Source: CAD feature listing. Evaluate the final solid. Frame: model axes, mm. Face numbers are marked on the shaded views. A direction names the side the tool comes from. Round coordinates to 2 decimals unless told otherwise and drop trailing zeros. Order: outer loops, then holes, each group sorted by start corner. A loop starts at its lowest first (then second) coordinate and runs counter-clockwise, first axis right, second up. Notation, with made-up numbers: (-24.75, -18.5) -> (28.25, -18.5) arc R7 cw to (28.25, -7.5) -> close; hole circle Ø5 at (2, 11). An arc over 180 degrees is marked (long way). Write item = value, one per line. Start each with the question number.
(1) Ray query, line 1 (Y direction, x = 30, z = 14.5); line 2 (Y direction, x = 30, z = 6); line 3 (Y direction, x = 0.5, z = 3). Return the intervals inside material, ascending.
(2) Contact query for flat-ended pins moving along their axis: pin 1 Ø9.5 at (x, y) = (0.5, -1.5) entering from +Z; pin 2 Ø10.5 at (x, y) = (-30, -30) entering from +Z; pin 3 Ø4 at (x, z) = (29, 38.5) entering from -Y; pin 4 Ø9 at (x, y) = (30, -30) entering from -Z. Output: stop coordinate, or through.
(3) Cut plane C-C on x = 30. Return the cut outline in (y, z), then the cut area to 3 significant figures.
(4) Draft query along Y for the marked faces 1, 2, 3 and 4. Return one class per face: released by +Y, released by -Y, zero draft, split by the parting line, or undercut.
(5) Cut plane D-D on y = 11. Return the cut outline in (x, z).
(6) Reachability of the marked faces 5, 6 and 7 from +Z, -Z, +X, -X, +Y, -Y: full face, straight path, thin tool, end or side. Return the list, or none.
(7) Cut plane A-A on y = 30. Return the cut outline in (x, z).
(8) Cut plane B-B on z = 9.5. Give the number of separate pieces and of enclosed holes in the cut face, then the cut area to 3 significant figures.
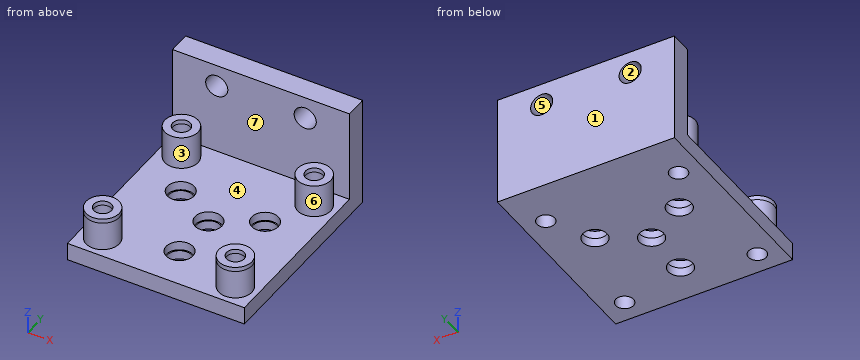
from build123d import *

# Parameters (mm, degrees)
F0_W      = 80
F0_H      = 80
F1_DEPTH  = 8
F2_R      = 6.05
F2_R_2    = 5.5
F3_DEPTH  = 4
F4_DEPTH  = 25
F5_DEPTH  = 25
F6_R      = 7.5
F6_R_2    = 4
F7_DEPTH  = 13
F8_DEPTH  = 25
F9_W      = 80
F9_H      = 10
F10_DEPTH = 50
F11_R     = 5
F12_DEPTH = 25
F13_DEPTH = 2


with BuildPart() as f1:
    # F0 (on Top) → F1 (new body)
    with BuildSketch(Plane.XY):
        Rectangle(F0_W, F0_H)
    extrude(amount=F1_DEPTH)

    # F2 (on face) → F3 (cut)
    with BuildSketch(Plane.XY.offset(8)):
        with Locations((-19.0525588833, 11)):
            Circle(F2_R)
        with Locations((-19.0525588833, 11)):
            Circle(F2_R_2, mode=Mode.SUBTRACT)
        with Locations((19.0525588833, 11)):
            Circle(F2_R)
        with Locations((19.0525588833, 11)):
            Circle(F2_R_2, mode=Mode.SUBTRACT)
        Circle(F2_R)
        Circle(F2_R_2, mode=Mode.SUBTRACT)
        with Locations((0, -22)):
            Circle(F2_R)
        with Locations((0, -22)):
            Circle(F2_R_2, mode=Mode.SUBTRACT)
    extrude(amount=-F3_DEPTH, mode=Mode.SUBTRACT)

    # F4 (cut): faces of the model
    f4_faces = [f1.faces().sort_by_distance(p)[0] for p in [
        (-19.0525588833, 11, 8),
        (19.0525588833, 11, 8),
        (0, -22, 8),
    ]]
    extrude(f4_faces, amount=-F4_DEPTH, mode=Mode.SUBTRACT)

    # F5 (cut): a face of the model
    f5_faces = [f1.faces().sort_by_distance(p)[0] for p in [
        (0, 0, 8),
    ]]
    extrude(f5_faces, amount=-F5_DEPTH, mode=Mode.SUBTRACT)

    # F6 (on face) → F7 (join)
    with BuildSketch(Plane.XY.offset(8)):
        with Locations((-30, 30)):
            Circle(F6_R)
        with Locations((-30, 30)):
            Circle(F6_R_2, mode=Mode.SUBTRACT)
        with Locations((30, 30)):
            Circle(F6_R)
        with Locations((30, 30)):
            Circle(F6_R_2, mode=Mode.SUBTRACT)
        with Locations((30, -30)):
            Circle(F6_R)
        with Locations((30, -30)):
            Circle(F6_R_2, mode=Mode.SUBTRACT)
        with Locations((-30, -30)):
            Circle(F6_R)
        with Locations((-30, -30)):
            Circle(F6_R_2, mode=Mode.SUBTRACT)
    extrude(amount=F7_DEPTH)

    # F8 (cut): faces of the model
    f8_faces = [f1.faces().sort_by_distance(p)[0] for p in [
        (-30, 30, 8),
        (30, 30, 8),
        (-30, -30, 8),
        (30, -30, 8),
    ]]
    extrude(f8_faces, amount=-F8_DEPTH, mode=Mode.SUBTRACT)

    # F9 (on face) → F10 (join)
    with BuildSketch(Plane(origin=(0, 0, 0), x_dir=(1, 0, 0), z_dir=(0, 0, -1))):
        with Locations((0, -45)):
            Rectangle(F9_W, F9_H)
    extrude(amount=-F10_DEPTH)

    # F11 (on face) → F12 (cut)
    with BuildSketch(Plane(origin=(0, 50, 0), x_dir=(-1, 0, 0), z_dir=(0, 1, 0))):
        with Locations((-20, 40)):
            Circle(F11_R)
        with Locations((20, 40)):
            Circle(F11_R)
    extrude(amount=-F12_DEPTH, mode=Mode.SUBTRACT)

    # F13 (add): faces of the model
    f13_faces = [f1.faces().sort_by_distance(p)[0] for p in [
        (-37.2878679656, 30, 21),
        (-37.2878679656, -30, 21),
        (22.7121320344, -30, 21),
        (22.7121320344, 30, 21),
    ]]
    extrude(f13_faces, amount=F13_DEPTH)


solid = f1.part
Evaluation:
q1.line_1 = -37.5 to -34, -26 to -22.5, 22.5 to 26, 34 to 37.5, 40 to 50
q1.line_2 = -40 to -34, -26 to 26, 34 to 50
q1.line_3 = -40 to -27.48, -16.52 to -5.48, 5.48 to 50
q2.pin_1 = 8
q2.pin_2 = 23
q2.pin_3 = 40
q2.pin_4 = 0
q3.outline = (-40, 0) -> (-34, 0) -> (-34, 23) -> (-37.5, 23) -> (-37.5, 8) -> (-40, 8) -> close; (-26, 0) -> (26, 0) -> (26, 23) -> (22.5, 23) -> (22.5, 8) -> (-22.5, 8) -> (-22.5, 23) -> (-26, 23) -> close; (34, 0) -> (50, 0) -> (50, 50) -> (40, 50) -> (40, 8) -> (37.5, 8) -> (37.5, 23) -> (34, 23) -> close
q3.area = 1,220 mm^2
q4.face_1 = released by +Y
q4.face_2 = zero draft
q4.face_3 = undercut
q4.face_4 = undercut
q5.outline = (-40, 0) -> (-24.55, 0) -> (-24.55, 4) -> (-25.1, 4) -> (-25.1, 8) -> (-40, 8) -> close; (-13.55, 0) -> (13.55, 0) -> (13.55, 4) -> (13, 4) -> (13, 8) -> (-13, 8) -> (-13, 4) -> (-13.55, 4) -> close; (24.55, 0) -> (40, 0) -> (40, 8) -> (25.1, 8) -> (25.1, 4) -> (24.55, 4) -> close
q6.face_5 = +Y, -Y
q6.face_6 = +Z
q6.face_7 = +Z, +X, -X
q7.outline = (-40, 0) -> (-34, 0) -> (-34, 23) -> (-37.5, 23) -> (-37.5, 8) -> (-40, 8) -> close; (-26, 0) -> (26, 0) -> (26, 23) -> (22.5, 23) -> (22.5, 8) -> (-22.5, 8) -> (-22.5, 23) -> (-26, 23) -> close; (34, 0) -> (40, 0) -> (40, 8) -> (37.5, 8) -> (37.5, 23) -> (34, 23) -> close
q8.separate_pieces = 5
q8.enclosed_holes = 4
q8.area = 1,310 mm^2
